Geometry check sheet. Reference: the model listing, model coordinates, mm. Round coordinates to 2 decimals unless told otherwise and drop trailing zeros. Order: outer loops, then holes, each group sorted by start corner. A loop starts at its lowest first (then second) coordinate and runs counter-clockwise, first axis right, second up.
(1) Cross-section at A-A on z = 0. Enter the section's corners in (x, y) (3 decimals).
(2) Thickness scan on L1, parallel to Z at x = 0, y = -3.1 (3 decimals); L2, parallel to X at y = -2.25, z = 1; L3, parallel to X at y = -2.9, z = -0.25. Record the ranges inside material, lowest first.
(3) Draft check along Z on faces 1 (the face through (2, 0, -2)), 2 (the face through (-2.38, -2.48, -10.74)), 3 (the face through (-1.13, -2.48, -0.87)). Enter one of: pulls with the +Z half, pulls with the -Z half, needs draft (parallel to the pull), parting line crosses it, or undercut.
(4) Gauge pin test, flat ends, axial feed: P1, Ø1, axis at x = -7.5, y = -2, coming from the +Z side; P2, Ø1.5, axis at y = -2.5, z = -1.5, coming from the -X side; P3, Ø4.5, axis at x = 0, z = 0, coming from the +Y side. Record the tip position at first contact, or that the pin passes through.
(5) Cross-section at B-B on x = 0. Enter the section's corners in (y, z) (3 decimals), and give its area (3 significant figures).
(6) Cross-section at C-C on y = -3.5. Enter the section's corners in (x, z) (3 decimals).
from build123d import *

# Parameters (mm, degrees)
F0_R     = 11
F0_R_2   = 1.425
F1_DEPTH = 5
F2_R     = 1
F3_R     = 1
F4_R     = 1
F5_R     = 1


with BuildPart() as f1:
    # F0 (on Front) → F1 (new body)
    with BuildSketch(Plane.XZ):
        Circle(F0_R)
        Circle(F0_R_2, mode=Mode.SUBTRACT)
    extrude(amount=F1_DEPTH)

    # F2
    f2_edges = [f1.edges().sort_by_distance(p)[0] for p in [
        (-1.425, -5, 0),
    ]]
    fillet(f2_edges, radius=F2_R)

    # F3
    f3_edges = [f1.edges().sort_by_distance(p)[0] for p in [
        (-1.425, 0, 0),
    ]]
    fillet(f3_edges, radius=F3_R)

    # F4
    f4_edges = [f1.edges().sort_by_distance(p)[0] for p in [
        (-11, -5, 0),
    ]]
    fillet(f4_edges, radius=F4_R)

    # F5
    f5_edges = [f1.edges().sort_by_distance(p)[0] for p in [
        (-11, 0, 0),
    ]]
    fillet(f5_edges, radius=F5_R)


solid = f1.part
Found:
1. outline: (-11, -4) arc R1 ccw to (-10, -5) - (-2.425, -5) arc R1 ccw to (-1.425, -4) - (-1.425, -1) arc R1 ccw to (-2.425, 0) - (-10, 0) arc R1 ccw to (-11, -1) - close; (1.425, -4) arc R1 ccw to (2.425, -5) - (10, -5) arc R1 ccw to (11, -4) - (11, -1) arc R1 ccw to (10, 0) - (2.425, 0) arc R1 ccw to (1.425, -1) - close
2. L1: z = -11 to -1.425, 1.425 to 11
2. L2: x = -10.95 to -1.02, 1.02 to 10.95
2. L3: x = -11 to -1.4, 1.4 to 11
3. face 1: needs draft
3. face 2: parting line crosses it
3. face 3: undercut
4. P1: stops at z = 8.49
4. P2: stops at x = -10.97
4. P3: stops at y = -0.02
5. outline: (-5, -10) arc R1 ccw to (-4, -11) - (-1, -11) arc R1 ccw to (0, -10) - (0, -2.425) arc R1 ccw to (-1, -1.425) - (-4, -1.425) arc R1 ccw to (-5, -2.425) - close; (-5, 2.425) arc R1 ccw to (-4, 1.425) - (-1, 1.425) arc R1 ccw to (0, 2.425) - (0, 10) arc R1 ccw to (-1, 11) - (-4, 11) arc R1 ccw to (-5, 10) - close
5. area: 94.0 mm2
6. outline: circle Ø22 at (0, 0); hole circle Ø2.85 at (0, 0)
